```python
from build123d import *

# Parameters (mm, degrees)
SKETCH1_R           = 2.5
BOSS_EXTRUDE1_DEPTH = 76
SKETCH2_W           = 20.5
SKETCH2_H           = 3
CUT_EXTRUDE1_DEPTH  = 70


with BuildPart() as part:
    # Sketch1 → Boss-Extrude1 (new body)
    with BuildSketch(Plane(origin=(0, 0, 0), x_dir=(0, 0, -1), z_dir=(1, 0, 0))):
        with BuildLine():
            Line((-24.25, -28.25), (24.25, -28.25))
            ThreePointArc((24.25, -28.25), (27.078427125, -27.078427125), (28.25, -24.25))
            Line((28.25, -24.25), (28.25, 24.25))
            ThreePointArc((28.25, 24.25), (27.078427125, 27.078427125), (24.25, 28.25))
            Line((24.25, 28.25), (-24.25, 28.25))
            ThreePointArc((-24.25, 28.25), (-27.078427125, 27.078427125), (-28.25, 24.25))
            Line((-28.25, 24.25), (-28.25, -24.25))
            ThreePointArc((-28.25, -24.25), (-27.078427125, -27.078427125), (-24.25, -28.25))
        make_face()
        with Locations((-23.55, 23.55)):
            Circle(SKETCH1_R, mode=Mode.SUBTRACT)
        with Locations((-23.55, -23.55)):
            Circle(SKETCH1_R, mode=Mode.SUBTRACT)
        with Locations((23.55, -23.55)):
            Circle(SKETCH1_R, mode=Mode.SUBTRACT)
        with Locations((23.55, 23.55)):
            Circle(SKETCH1_R, mode=Mode.SUBTRACT)
    extrude(amount=-BOSS_EXTRUDE1_DEPTH)

    # Sketch2 → Revolve1 (revolve)
    with BuildSketch(Plane(origin=(0, 0, 0), x_dir=(1, 0, 0), z_dir=(0, 1, 0))):
        with Locations((10.25, 1.5)):
            Rectangle(SKETCH2_W, SKETCH2_H)
    revolve(axis=Axis((0, 0, 0), (1, 0, 0)))

    # Sketch3 → Cut-Extrude1 (cut)
    with BuildSketch(Plane.ZY.offset(76)):
        with BuildLine():
            Line((-28.25, -16.25), (-28.25, -24.25))
            ThreePointArc((-28.25, -24.25), (-27.078427125, -27.078427125), (-24.25, -28.25))
            Line((-24.25, -28.25), (-16.25, -28.25))
            ThreePointArc((-16.25, -28.25), (-19.764718626, -19.764718626), (-28.25, -16.25))
        make_face()
        with BuildLine():
            Line((-16.25, 28.25), (-24.25, 28.25))
            ThreePointArc((-24.25, 28.25), (-27.078427125, 27.078427125), (-28.25, 24.25))
            Line((-28.25, 24.25), (-28.25, 16.25))
            ThreePointArc((-28.25, 16.25), (-19.764718626, 19.764718626), (-16.25, 28.25))
        make_face()
        with BuildLine():
            Line((28.25, 16.25), (28.25, 24.25))
            ThreePointArc((28.25, 24.25), (27.078427125, 27.078427125), (24.25, 28.25))
            Line((24.25, 28.25), (16.25, 28.25))
            ThreePointArc((16.25, 28.25), (19.764718626, 19.764718626), (28.25, 16.25))
        make_face()
        with BuildLine():
            Line((16.25, -28.25), (24.25, -28.25))
            ThreePointArc((24.25, -28.25), (27.078427125, -27.078427125), (28.25, -24.25))
            Line((28.25, -24.25), (28.25, -16.25))
            ThreePointArc((28.25, -16.25), (19.764718626, -19.764718626), (16.25, -28.25))
        make_face()
    extrude(amount=-CUT_EXTRUDE1_DEPTH, mode=Mode.SUBTRACT)


solid = part.part
```
Geometry: final body of the model. Coordinates: model frame, mm. A direction names the side the tool comes from. Coordinates: 2 decimals unless noted, no trailing zeros. Order: outer loops, then holes, each group sorted by start corner. A loop starts at its lowest first (then second) coordinate and runs counter-clockwise, first axis right, second up. Notation, with made-up numbers: (48.25, -39) -> (67.25, -39) arc R16 ccw to (67.25, -25) -> close; hole circle Ø11 at (26.5, 33.5). An arc over 180 degrees is marked (long way). Answer in a Markdown table with one row per item.
Item 1: Section D-D on z = -7.5. Output: boundary loops of the cut face in (x, y).
Return value:
| item | result |
|---|---|
| outline | (-76, -28.25) -> (0, -28.25) -> (0, 28.25) -> (-76, 28.25) -> close |
Item 2: Section C-C on z = -23. Output: boundary loops of the cut face in (x, y), plus the area to 3 significant figures.
Return value:
| item | result |
|---|---|
| outline | (-76, -17.46) -> (-6, -17.46) -> (-6, -21.11) -> (0, -21.11) -> (0, 21.11) -> (-6, 21.11) -> (-6, 17.46) -> (-76, 17.46) -> close; (-6, -28.25) -> (0, -28.25) -> (0, -25.99) -> (-6, -25.99) -> close; (-6, 25.99) -> (0, 25.99) -> (0, 28.25) -> (-6, 28.25) -> close |
| area | 2,720 mm² |
Item 3: Ray query, L1, parallel to Y at x = -4.2, z = 23.55; L2, parallel to X at y = -5, z = 10; L3, parallel to X at y = -24.5, z = 18. Return the intervals inside material, ascending.
Return value:
| item | result |
|---|---|
| L1 | y = -28.25 to -26.05, -21.05 to 21.05, 26.05 to 28.25 |
| L2 | x = -76 to 0 |
| L3 | x = -6 to 0 |
Item 4: Section B-B on y = 0. Output: boundary loops of the cut face in (x, z), plus the area to 3 significant figures.
Return value:
| item | result |
|---|---|
| outline | (-76, -28.25) -> (0, -28.25) -> (0, -3) -> (20.5, -3) -> (20.5, 3) -> (0, 3) -> (0, 28.25) -> (-76, 28.25) -> close |
| area | 4,420 mm² |
Item 5: Access query for faces 1 (the flat face through (-6, -20.8, -23.7)), 2 (the cylindrical face through (-41.49, 19.67, -19.86)), 3 (the flat face through (-37, 28.25, 0)), 4 (the flat face through (-6, 23.7, 20.8)). Directions: +Z, -Z, +X, -X, +Y, -Y. A direction counts if a zero-diameter tool reaches every point of the face in a straight line with its end or side. Return the directions, or none.
Return value:
| item | result |
|---|---|
| face 1 | -Z, -X, -Y |
| face 2 | -Z, -X, +Y |
| face 3 | +Z, -Z, +X, -X, +Y |
| face 4 | +Z, -X, +Y |
Item 6: Contact query for flat-ended pins moving along their axis: P1, Ø6.5, axis at y = -23.55, z = -23.55, coming from the +X side; P2, Ø3, axis at x = -58, z = -19.5, coming from the -Y side; P3, Ø6, axis at y = 23.55, z = -23.55, coming from the -X side; P4, Ø4.5, axis at y = 23.55, z = 23.55, coming from the -X side. Output: stop coordinate, or through.
Return value:
| item | result |
|---|---|
| P1 | stops at x = 0 |
| P2 | stops at y = -22.01 |
| P3 | stops at x = -6 |
| P4 | passes through |
Item 7: Draft query along Y for faces 5 (the flat face through (-6, -20.8, 23.5)), 6 (the cylindrical face through (-2.96, -25.99, 24.09)), 7 (the cylindrical face through (-41.49, -19.67, 19.86)). Return one class per face: released by +Y, released by -Y, zero draft, split by the parting line, or undercut.
Return value:
| item | result |
|---|---|
| face 5 | zero draft |
| face 6 | undercut |
| face 7 | released by -Y |
Item 8: Section A-A on x = -42.5. Output: boundary loops of the cut face in (y, z), plus the area to 3 significant figures.
Return value:
| item | result |
|---|---|
| outline | (-28.25, -16.25) arc R12 cw to (-16.25, -28.25) -> (16.25, -28.25) arc R12 cw to (28.25, -16.25) -> (28.25, 16.25) arc R12 cw to (16.25, 28.25) -> (-16.25, 28.25) arc R12 cw to (-28.25, 16.25) -> close |
| area | 2,740 mm² |
